Autodesk Fusion 360 part; units mm, degrees
sketch "草图1" plane through (0, 0, 0) normal (0, 0, 1) x (1, 0, 0)
  circle A0 centre (0, 0) radius 1.5
  circle A1 centre (-14, 0) radius 1.5
  line L0 (-14, 0) -> (0, 0) construction
  line L1 (-7, 0) -> (-7, -17.5669) construction
  dimension "d1" = 3
  dimension "d2" = 14
  dimension "d3" = 3
sketch "草图2" plane through (0, 0, 0) normal (0, 0, 1) x (1, 0, 0)
  line L0 (-17.3282, -10.7) -> (-17.3282, 3)
  line L1 (-17.3282, 3) -> (3.3282, 3)
  line L2 (3.3282, 3) -> (3.3282, -10.7)
  line L3 (-7, 0) -> (-7, -17.5669)
  line L4 (3.3282, -10.7) -> (-17.3282, -10.7)
  line L5 (-14, 0) -> (0, 0)
  dimension "d4" = 10.7
  dimension "d11" = 3
extrude "拉伸1" add sketch "草图2" along normal blind 1.5 in component "Component'"
extrude "拉伸2" cut sketch "草图1" along normal blind 4 in component "Component'"
sketch "草图4" plane through (0, 0, 1.5) normal (0, 0, 1) x (-1, 0, 0)
  circle A0 centre (14, 0) radius 1.5
  circle A1 centre (0, 0) radius 1.5
  line L0 (-3.3282, 10.7) -> (-3.3282, -3)
  line L1 (-3.3282, -3) -> (17.3282, -3)
  line L2 (17.3282, -3) -> (17.3282, 10.7)
  line L3 (17.3282, 10.7) -> (-3.3282, 10.7)
  line L4 (-3.3282, 10.7) -> (-3.3282, 7.7)
  line L5 (-3.3282, 7.7) -> (17.3282, 7.7)
  line L6 (17.3282, 10.7) -> (-3.3282, 10.7)
  dimension "d12" = 3
extrude "拉伸3" add sketch "草图4" along normal blind 7.5 contours L0 L2 L3 L4 L5 L6 in component "Component'"
sketch "草图5" plane through (0, -7.7, 0) normal (0, 1, 0) x (-1, 0, 0)
  line L0 (-3.3282, 1.5) -> (17.3282, 1.5)
  line L1 (17.3282, 1.5) -> (17.3282, 9)
  line L2 (17.3282, 9) -> (-3.3282, 9)
  line L3 (-3.3282, 9) -> (-3.3282, 1.5)
  line L4 (-3.3282, 6.5) -> (17.3282, 6.5)
  line L5 (17.3282, 9) -> (-3.3282, 9)
  dimension "d15" = 2.5
extrude "拉伸4" add sketch "草图5" along normal blind 6.5 contours L1 L2 L3 L4 L5 in component "Component'"
sketch "草图6" plane through (-17.3282, 0, 0) normal (-1, 0, 0) x (0, -1, 0)
  line L0 (-3, 0) -> (10.7, 0)
  line L1 (10.7, 0) -> (10.7, 9)
  line L2 (10.7, 9) -> (1.2, 9)
  line L3 (1.2, 9) -> (1.2, 6.5)
  line L4 (1.2, 6.5) -> (7.7, 6.5)
  line L5 (7.7, 6.5) -> (7.7, 1.5)
  line L6 (7.7, 1.5) -> (-3, 1.5)
  line L7 (-3, 1.5) -> (-3, 0)
  circle A0 centre (4.7, 7.6) radius 1.05
  point P0 (4.7, 7.6)
  dimension "d18" = 3
  dimension "d19" = 6.1
  dimension "d20" = 2.1
extrude "拉伸5" cut sketch "草图6" against normal blind 8.2 contours A0 in component "Component'"
component "Component'" placed x (1, 0, 0) y (0, 1, 0) z (0, 0, 1) at (0, 0, 0)
Design review of the part built by this model. Coordinates are the model's own, in mm. A direction names the side the tool comes from. Give positions to 0.01 mm unless a question says otherwise; leave off trailing zeros. Loops run counter-clockwise (first coordinate to the right, second up) from the corner with the lowest first, then second, coordinate; pieces in that order, holes last. Notation, with made-up numbers: (-29, 58.5) -> (-15, 58.5) arc R27 ccw to (-15, 93.5) -> close; hole circle Ø9 at (27.5, 82.25). An arc over 180 degrees is marked (long way). One line per item, written item: value.
Q1. We need section C-C on y = 0. Give the boundary of the cut face in (x, z), and give its area (3 significant figures).
Numbers:
outline: (-17.33, 0) -> (-15.5, 0) -> (-15.5, 1.5) -> (-17.33, 1.5) -> close; (-12.5, 0) -> (-1.5, 0) -> (-1.5, 1.5) -> (-12.5, 1.5) -> close; (1.5, 0) -> (3.33, 0) -> (3.33, 1.5) -> (1.5, 1.5) -> close
area: 22.0 mm^2
Q2. We need section B-B on x = -16. Give the boundary of the cut face in (y, z), and give its area (3 significant figures).
Numbers:
outline: (-10.7, 0) -> (3, 0) -> (3, 1.5) -> (-7.7, 1.5) -> (-7.7, 6.5) -> (-1.2, 6.5) -> (-1.2, 9) -> (-10.7, 9) -> close; hole circle Ø2.1 at (-4.7, 7.6)
area: 55.8 mm^2
Q3. We need section D-D on z = 7.6. Give the boundary of the cut face in (x, y), and give its area (3 significant figures).
Numbers:
outline: (-17.33, -10.7) -> (3.33, -10.7) -> (3.33, -1.2) -> (-17.33, -1.2) -> (-17.33, -3.65) -> (-9.13, -3.65) -> (-9.13, -5.75) -> (-17.33, -5.75) -> close
area: 179 mm^2
Q4. We need section A-A on y = -4.7. Give the boundary of the cut face in (x, z), and give its area (3 significant figures).
Numbers:
outline: (-17.33, 0) -> (3.33, 0) -> (3.33, 1.5) -> (-17.33, 1.5) -> close; (-17.33, 6.5) -> (3.33, 6.5) -> (3.33, 9) -> (-17.33, 9) -> (-17.33, 8.65) -> (-9.13, 8.65) -> (-9.13, 6.55) -> (-17.33, 6.55) -> close
area: 65.4 mm^2
Q5. Machinability: for faces 5 (the flat face through (-7, -1.2, 8)), 6 (the flat face through (3.328, -7, 7)), 7 (the cylindrical face through (-15.5, -0.07, 0.74)), 8 (the flat face through (-7, -7.7, 4)), which of the approach directions +Z, -Z, +X, -X, +Y, -Y give a long, thin tool a straight path to every point of the face, cutting with its end or side? Answer none if there is none.
Numbers:
face 5: +Z, +X, -X, +Y
face 6: +Z, -Z, +X, +Y, -Y
face 7: -Z
face 8: +X, -X, +Y
Q6. For pin 1 Ø1.5 at (x, z) = (-6.5, 5) entering from +Y; pin 2 Ø0.8 at (x, z) = (-11, 7.5) entering from +Y; pin 3 Ø1 at (y, z) = (-5, 7.5) entering from -X, all flat-tipped, find the tip position at first contact; note any pin that passes through.
Numbers:
pin 1: stops at y = -7.7
pin 2: stops at y = -1.2
pin 3: stops at x = -9.13
Q7. Draft analysis for pull direction Z (two halves, no side actions). For faces 1 (the flat face through (-17.328, -5, 1)), 2 (the cylindrical face through (-13.286, -3.926, 8.31)), 3 (the flat face through (-7, -4, 0)), 4 (the flat face through (-9.128, -5, 8)), state which applies: pulls with the +Z half, pulls with the -Z half, needs draft (parallel to the pull), parting line crosses it, or undercut.
Numbers:
face 1: needs draft
face 2: undercut
face 3: pulls with the -Z half
face 4: undercut
Q8. For L1, parallel to X at y = 0, z = 0.65; L2, parallel to Z at x = -7.25, y = -3.25; L3, parallel to Y at x = 0, z = 0.8, list the stretches that pass through material, from the lowest coordinate up.
Numbers:
L1: x = -17.33 to -15.5, -12.5 to -1.5, 1.5 to 3.33
L2: z = 0 to 1.5, 6.5 to 9
L3: y = -10.7 to -1.5, 1.5 to 3
